from build123d import *

# Parameters (mm, degrees)
F1_DEPTH = 50
F2_R     = 11.5
F2_R_2   = 1.85
F3_DEPTH = 3
F4_SIZE  = 6
F6_DEPTH = 3


with BuildPart() as f1:
    # F0 (on Right) → F1 (new body)
    with BuildSketch(Plane.YZ):
        with BuildLine():
            Line((-52, 3), (-52, 0))
            Line((-52, 0), (-2.5, 0))
            ThreePointArc((-2.5, 0), (-0.732233, 0.732233), (0, 2.5))
            Line((0, 2.5), (0, 52))
            Line((0, 52), (-3, 52))
            Line((-3, 52), (-3, 3))
            Line((-3, 3), (-52, 3))
        make_face()
    extrude(amount=-F1_DEPTH)

    # F2 (on Top) → F3 (cut)
    with BuildSketch(Plane.XY):
        with Locations((-25, -31)):
            Circle(F2_R)
        with Locations((-9.5, -46.5)):
            Circle(F2_R_2)
        with Locations((-9.5, -15.5)):
            Circle(F2_R_2)
        with Locations((-40.5, -46.5)):
            Circle(F2_R_2)
        with Locations((-40.5, -15.5)):
            Circle(F2_R_2)
    extrude(amount=F3_DEPTH, mode=Mode.SUBTRACT)

    # F4
    f4_edges = [f1.edges().sort_by_distance(p)[0] for p in [
        (0, -52, 1.5),
        (-50, -52, 1.5),
        (0, -1.5, 52),
        (-50, -1.5, 52),
    ]]
    chamfer(f4_edges, length=F4_SIZE)

    # F5 (on face) → F6 (cut)
    with BuildSketch(Plane(origin=(0, 0, 0), x_dir=(-1, 0, 0), z_dir=(0, 1, 0))):
        with BuildLine():
            Line((39.5, 11), (39.5, 41))
            ThreePointArc((39.5, 41), (37.5, 43), (35.5, 41))
            Line((35.5, 41), (35.5, 11))
            ThreePointArc((35.5, 11), (37.5, 9), (39.5, 11))
        make_face()
        with BuildLine():
            ThreePointArc((14.5, 41), (12.5, 43), (10.5, 41))
            Line((10.5, 41), (10.5, 11))
            ThreePointArc((10.5, 11), (12.5, 9), (14.5, 11))
            Line((14.5, 11), (14.5, 41))
        make_face()
    extrude(amount=-F6_DEPTH, mode=Mode.SUBTRACT)


solid = f1.part
Part model, mm, in its own coordinate system. A direction names the side the tool comes from. Coordinates: 2 decimals unless noted, no trailing zeros. Write each loop counter-clockwise with the first axis right and the second up, starting at its lowest first coordinate (ties: lowest second). Pieces come first, ordered by that corner, then holes. Notation, with made-up numbers: M -20.75,17.5 L 27.25,17.5 A30 ccw 27.25,54.5 Z; hole C 30,-13.75 d1. An arc over 180 degrees is marked long. Return JSON: item names as keys, results as strings.
1. Flat gauge pins, fed straight in: pin 1 Ø2 at (x, y) = (-40.5, -15.5) entering from -Z; pin 2 Ø4.5 at (x, y) = (-40.5, -46.5) entering from +Z. Where does each tip first touch, or does it go through?
Determined:
{"pin 1": "through", "pin 2": "z = 3"}
2. Saw through at C-C, the plane z = 17.5. Write the cut outline in (x, y).
Determined:
{"outline": "M -50,-3 L -39.5,-3 L -39.5,0 L -50,0 Z; M -35.5,-3 L -14.5,-3 L -14.5,0 L -35.5,0 Z; M -10.5,-3 L 0,-3 L 0,0 L -10.5,0 Z"}
3. Saw through at D-D, the plane x = -9.5. Write the cut outline in (y, z).
Determined:
{"outline": "M -52,0 L -48.35,0 L -48.35,3 L -52,3 Z; M -44.65,0 L -17.35,0 L -17.35,3 L -44.65,3 Z; M -13.65,0 L -2.5,0 A2.5 ccw 0,2.5 L 0,52 L -3,52 L -3,3 L -13.65,3 Z"}
4. Saw through at A-A, the plane x = -25. Write the cut outline in (y, z).
Determined:
{"outline": "M -52,0 L -42.5,0 L -42.5,3 L -52,3 Z; M -19.5,0 L -2.5,0 A2.5 ccw 0,2.5 L 0,52 L -3,52 L -3,3 L -19.5,3 Z"}
5. 3-axis set-ups, long thin cutter, end or side, ignore diameter. For faces 1 (the face through (-25, -3, 28)), 2 (the face through (-37.5, -1.5, 43)), 3 (the face through (-50, -12.9, 2.7)): which of +Z, -Z, +X, -X, +Y, -Y reach the whole face in a straight line?
Determined:
{"face 1": "+Z, +X, -X, -Y", "face 2": "+Y, -Y", "face 3": "+Z, -Z, -X, +Y, -Y"}
6. Pull direction Z, two halves, no side cores. Call faces 4 (the face through (-25, -16, 3)), 5 (the face through (-10.5, -1, 26)), 6 (the face through (-24.65, -0.752, 0.713)): pulls with the +Z half, pulls with the -Z half, needs draft (parallel to the pull), parting line crosses it, or undercut.
Determined:
{"face 4": "pulls with the +Z half", "face 5": "undercut", "face 6": "pulls with the -Z half"}
7. Probe L1, parallel to Y at x = -40.5, z = 2.45; L2, parallel to Z at x = -42, y = -4; L3, parallel to Y at x = -2.5, z = 16.5. List the from-to ranges inside material, lowest first.
Determined:
{"L1": "-52 to -48.35, -44.65 to -17.35, -13.65 to 0", "L2": "0 to 3", "L3": "-3 to 0"}
8. Saw through at B-B, the plane y = -29. Write the cut outline in (x, z).
Determined:
{"outline": "M -50,0 L -36.32,0 L -36.32,3 L -50,3 Z; M -13.68,0 L 0,0 L 0,3 L -13.68,3 Z"}
